The drawing under review shows one solid part. Ordinate dimensions are in mm from its lowest x, y, z. Round coordinates to 2 decimals unless told otherwise and drop trailing zeros. Loops run counter-clockwise (first coordinate to the right, second up) from the corner with the lowest first, then second, coordinate; pieces in that order, holes last. Notation, with made-up numbers: (-18.75, 17.25) - (-9.75, 17.25) arc R16 ccw to (-9.75, 27.25) - close; hole circle Ø2 at (88, -34). An arc over 180 degrees is marked (long way). Answer as CSV lines item,"result".
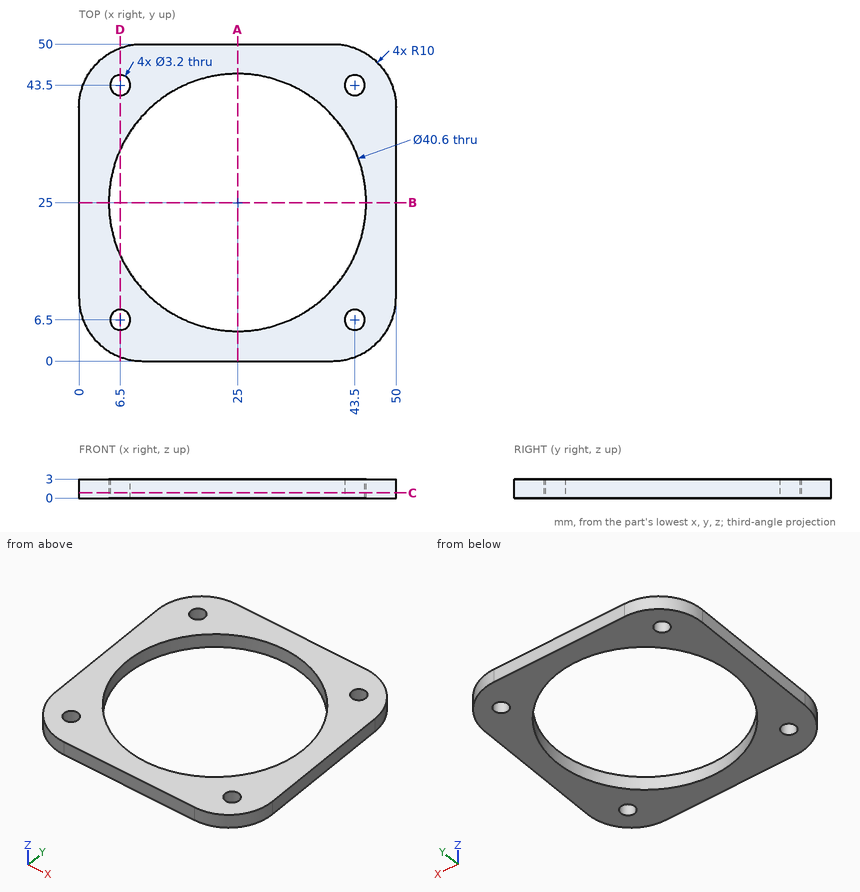
1. Clearance check with a flat-ended pin moving along its axis: pin 1 (1 mm diameter, centred on x = 8, z = 1.5, fed in from +Y). State where the tip first meets the part, or that it passes through.
Numbers:
pin 1,"stops at y = 49.89"
2. Take a section at D-D (x = 6.5). State the section outline as (y, z) points, plus the area to 3 significant figures.
Numbers:
outline,"(0.63, 0) - (4.9, 0) - (4.9, 3) - (0.63, 3) - close; (8.1, 0) - (16.64, 0) - (16.64, 3) - (8.1, 3) - close; (33.36, 0) - (41.9, 0) - (41.9, 3) - (33.36, 3) - close; (45.1, 0) - (49.37, 0) - (49.37, 3) - (45.1, 3) - close"
area,"76.9 mm²"
3. Take a section at A-A (x = 25). State the section outline as (y, z) points, plus the area to 3 significant figures.
Numbers:
outline,"(0, 0) - (4.7, 0) - (4.7, 3) - (0, 3) - close; (45.3, 0) - (50, 0) - (50, 3) - (45.3, 3) - close"
area,"28.2 mm²"
4. Wall thickness on probe 1 along Y at (x, z) = (25, 1.3); probe 2 along Y at (x, z) = (43.5, 0.9); probe 3 along X at (y, z) = (26.5, 2.7): over which ranges is each line inside the solid? List them lowest first.
Numbers:
probe 1,"y = 0 to 4.7, 45.3 to 50"
probe 2,"y = 0.63 to 4.9, 8.1 to 16.64, 33.36 to 41.9, 45.1 to 49.37"
probe 3,"x = 0 to 4.76, 45.24 to 50"
5. Take a section at C-C (z = 0.8). State the section outline as (x, y) points, plus the area to 3 significant figures.
Numbers:
outline,"(0, 10) arc R10 ccw to (10, 0) - (40, 0) arc R10 ccw to (50, 10) - (50, 40) arc R10 ccw to (40, 50) - (10, 50) arc R10 ccw to (0, 40) - close; hole circle Ø40.6 at (25, 25); hole circle Ø3.2 at (6.5, 6.5); hole circle Ø3.2 at (6.5, 43.5); hole circle Ø3.2 at (43.5, 6.5); hole circle Ø3.2 at (43.5, 43.5)"
area,"1,090 mm²"
